from build123d import *

# Parameters (mm, degrees)
BOSS_EXTRUDE1_DEPTH = 20
SKETCH2_W           = 20
SKETCH2_H           = 20
BOSS_EXTRUDE2_DEPTH = 220
BOSS_EXTRUDE3_DEPTH = 20
LPATTERN1_COUNT     = 2
LPATTERN1_PITCH     = 84.5


with BuildPart() as part:
    # Sketch1 → Boss-Extrude1 (new body)
    with BuildSketch(Plane.XY):
        Polygon((0, 0), (350, 350), (350, 0), (330, 0), (330, 301.715728753), (28.284271247, 0), align=None)
    boss_extrude1 = extrude(amount=BOSS_EXTRUDE1_DEPTH)

    # Sketch2 → Boss-Extrude2 (add)
    with BuildSketch(Plane.XY.offset(20)):
        with Locations((340, 80)):
            Rectangle(SKETCH2_W, SKETCH2_H)
        Polygon((98.284271247, 70), (112.426406871, 84.142135624), (98.284271247, 98.284271247), (84.142135624, 84.142135624), align=None)
    extrude(amount=BOSS_EXTRUDE2_DEPTH)

    # Mirror1: Boss-Extrude1 across plane
    add(boss_extrude1.mirror(Plane(origin=(0, 0, 130), x_dir=(1, 0, 0), z_dir=(0, 0, -1))))

    # Sketch5 → Boss-Extrude3 (add)
    with BuildSketch(Plane.XY.offset(182.25)):
        Polygon((330, 70), (98.284271247, 70), (118.284271247, 90), (330, 90), align=None)
    boss_extrude3 = extrude(amount=-BOSS_EXTRUDE3_DEPTH)

    # LPattern1: Boss-Extrude3 ×2
    with Locations(*[(0, 0, -i * LPATTERN1_PITCH) for i in range(1, LPATTERN1_COUNT)]):
        add(boss_extrude3)


solid = part.part
Can you work these out from the model? Positions are in its coordinate system, mm. A direction names the side the tool comes from. Round coordinates to 2 decimals unless told otherwise and drop trailing zeros. Order: outer loops, then holes, each group sorted by start corner. A loop starts at its lowest first (then second) coordinate and runs counter-clockwise, first axis right, second up. Notation, with made-up numbers: (28.25, 4.5) - (78.25, 4.5) arc R6 ccw to (78.25, 9.5) - close; hole circle Ø9 at (54.5, 10). An arc over 180 degrees is marked (long way). Answer in a Markdown table with one row per item.
(1) Suppose I cut it at C-C, the plane y = 129. Please give me the cut outline in (x, z).
From the geometry:
| item | result |
|---|---|
| outline | (129, 0) - (157.28, 0) - (157.28, 20) - (129, 20) - close; (129, 240) - (157.28, 240) - (157.28, 260) - (129, 260) - close; (330, 0) - (350, 0) - (350, 20) - (330, 20) - close; (330, 240) - (350, 240) - (350, 260) - (330, 260) - close |
(2) Suppose I cut it at B-B, the plane x = 310.5. Please give me the cut outline in (y, z).
From the geometry:
| item | result |
|---|---|
| outline | (70, 77.75) - (90, 77.75) - (90, 97.75) - (70, 97.75) - close; (70, 162.25) - (90, 162.25) - (90, 182.25) - (70, 182.25) - close; (282.22, 0) - (310.5, 0) - (310.5, 20) - (282.22, 20) - close; (282.22, 240) - (310.5, 240) - (310.5, 260) - (282.22, 260) - close |
(3) Suppose I cut it at A-A, the plane z = 188.5. Please give me the cut outline in (x, y), plus the area to 3 significant figures.
From the geometry:
| item | result |
|---|---|
| outline | (84.14, 84.14) - (98.28, 70) - (112.43, 84.14) - (98.28, 98.28) - close; (330, 70) - (350, 70) - (350, 90) - (330, 90) - close |
| area | 800 mm2 |
(4) Suppose I cut it at D-D, the plane x = 36. Please give me the cut outline in (y, z).
From the geometry:
| item | result |
|---|---|
| outline | (7.72, 0) - (36, 0) - (36, 20) - (7.72, 20) - close; (7.72, 240) - (36, 240) - (36, 260) - (7.72, 260) - close |
(5) For P1, Ø10, axis at x = 200.5, y = 76.5, coming from the -Z side; P2, Ø16, axis at x = 241.5, y = 78.5, coming from the +Z side; P3, Ø1, axis at y = 72, z = 59, coming from the -X side, each with a flat end and sliding along its axis, tell me the tip position at first contact or that it passes through.
From the geometry:
| item | result |
|---|---|
| P1 | stops at z = 77.75 |
| P2 | stops at z = 182.25 |
| P3 | stops at x = 95.78 |
(6) Please list where these lines run through material, in increasing order: L1, parallel to Z at x = 259.5, y = 246; L2, parallel to Y at x = 320.5, z = 167; L3, parallel to X at y = 165, z = 247.5. Write a range as from..to.
From the geometry:
| item | result |
|---|---|
| L1 | z = 0..20, 240..260 |
| L2 | y = 70..90 |
| L3 | x = 165..193.28, 330..350 |
(7) If we mould it in two halves opening along X, with no side actions, what happens to faces 4 (the face through (105.454, 91.114, 128.46)), 5 (the face through (91.114, 77.17, 128.46)), 6 (the face through (14, 0, 10))? For each: released by +X, released by -X, zero draft, split by the parting line, or undercut.
From the geometry:
| item | result |
|---|---|
| face 4 | undercut |
| face 5 | released by -X |
| face 6 | zero draft |
(8) Which directions (+Z, -Z, +X, -X, +Y, -Y) give clear straight access to the entire face, cutting with the end or side of a thin tool? Please do faces 1 (the face through (330, 139, 244)), 2 (the face through (340, 35, 20)), 3 (the face through (168.671, 140.387, 13.14)).
From the geometry:
| item | result |
|---|---|
| face 1 | +Z, -Y |
| face 2 | +X, -X, -Y |
| face 3 | -Z, -Y |
